Check sheet for the modelled part. Datum: model origin and axes. Units: mm. A direction names the side the tool comes from. Coordinates: 2 decimals unless noted, no trailing zeros. Loops run counter-clockwise (first coordinate to the right, second up) from the corner with the lowest first, then second, coordinate; pieces in that order, holes last. Notation, with made-up numbers: M -40,13.25 L -4,13.25 A28 ccw -4,45.25 Z; hole C 62,19 d1. An arc over 180 degrees is marked long. Write each question's results on one line, items separated by ' | '. Start each with the question number.
from build123d import *

# Parameters (mm, degrees)
PAD_DEPTH         = 10
SKETCH001_W       = 20.5
SKETCH001_H       = 6.5
POCKET_DEPTH      = 8
SKETCH002_W       = 20.5
SKETCH002_H       = 4
POCKET001_DEPTH   = 5
POCKET002_DEPTH   = 5
POCKET002_FACE1_W = 10
POCKET002_FACE1_H = 34
PAD001_DEPTH      = 1
PAD001_FACE3_W    = 10
PAD001_FACE3_H    = 10
PAD002_DEPTH      = 1


with BuildPart() as part:
    # Sketch → Pad (new body)
    with BuildSketch(Plane.XZ):
        Polygon((0, 10), (24, 10), (24, 2), (34, 2), (34, 0), (0, 0), align=None)
    extrude(amount=PAD_DEPTH)

    # Sketch001 (on Face7 of Pad) → Pocket (cut)
    with BuildSketch(Plane(origin=(0, 0, 0), x_dir=(1, 0, 0), z_dir=(0, 1, 0))):
        with Locations((11.75, -5.25)):
            Rectangle(SKETCH001_W, SKETCH001_H)
    extrude(amount=-POCKET_DEPTH, mode=Mode.SUBTRACT)

    # Sketch002 (on Face13 of Pocket) → Pocket001 (cut)
    with BuildSketch(Plane(origin=(0, -8, 0), x_dir=(1, 0, 0), z_dir=(0, 1, 0))):
        with Locations((11.75, -5.25)):
            Rectangle(SKETCH002_W, SKETCH002_H)
    extrude(amount=-POCKET001_DEPTH, mode=Mode.SUBTRACT)

    # Sketch003 (on Face6 of Pocket001) → Pocket002 (cut)
    with BuildSketch(Plane(origin=(0, 0, 2), x_dir=(-1, 0, 0), z_dir=(0, 0, 1))):
        with BuildLine():
            ThreePointArc((-30, 4.05), (-31.55, 2.5), (-30, 0.95))
            Line((-30, 0.95), (-26, 0.95))
            ThreePointArc((-26, 0.95), (-24.45, 2.5), (-26, 4.05))
            Line((-26, 4.05), (-30, 4.05))
        make_face()
    extrude(amount=-POCKET002_DEPTH, mode=Mode.SUBTRACT)

    # Pocket002 Face1 → Pad001 (add)
    with BuildSketch(Plane(origin=(16.314411, -5.155816, 0), x_dir=(0, -1, 0), z_dir=(0, 0, -1))):
        with Locations((-0.155816, -0.685589)):
            Rectangle(POCKET002_FACE1_W, POCKET002_FACE1_H)
        with BuildLine():
            Line((-1.105816, -9.685589), (-1.105816, -13.685589))
            ThreePointArc((-1.105816, -13.685589), (-2.655816, -15.235589), (-4.205816, -13.685589))
            Line((-4.205816, -13.685589), (-4.205816, -9.685589))
            ThreePointArc((-4.205816, -9.685589), (-2.655816, -8.135589), (-1.105816, -9.685589))
        make_face(mode=Mode.SUBTRACT)
    extrude(amount=PAD001_DEPTH)

    # Pad001 Face3 → Pad002 (add)
    with BuildSketch(Plane(origin=(29.249183, -5.622957, 2), x_dir=(0, 1, 0), z_dir=(0, 0, 1))):
        with Locations((0.622957, 0.249183)):
            Rectangle(PAD001_FACE3_W, PAD001_FACE3_H)
        with BuildLine():
            ThreePointArc((4.672957, -0.750817), (3.122957, -2.300817), (1.572957, -0.750817))
            Line((1.572957, -0.750817), (1.572957, 3.249183))
            ThreePointArc((1.572957, 3.249183), (3.122957, 4.799183), (4.672957, 3.249183))
            Line((4.672957, 3.249183), (4.672957, -0.750817))
        make_face(mode=Mode.SUBTRACT)
    extrude(amount=PAD002_DEPTH)


solid = part.part
Item 1: Section check C-C (x = 16.5). Record the cut outline in (y, z), plus the area to 3 significant figures.
Item 2: Thickness scan on line 1 (Z direction, x = 5, y = -1.5); line 2 (X direction, y = -4.5, z = 6.25); line 3 (X direction, y = -6.5, z = 2.5). Record the ranges inside material, lowest first.
Item 3: Depth check by flat-ended pin: P1, Ø3, axis at x = 26.5, y = -2.5, coming from the +Z side; P2, Ø3.5, axis at y = -4, z = 8, coming from the +X side; P3, Ø1, axis at x = 25.5, y = -5, coming from the +Z side. Enter the tip coordinate at first touch or a pass-through.
Item 4: Section check B-B (z = 5). Record the cut outline in (x, y), plus the area to 3 significant figures.
Item 5: Tool access check on faces 1 (the face through (24, -5, 7)), 2 (the face through (12, -4, 8.5)), 3 (the face through (28, -0.95, 1)). Record the directions out of +Z, -Z, +X, -X, +Y, -Y that give a thin tool (end or side, any length) a straight path to the whole face; none if there is none.
Item 6: Section check D-D (y = -8.75). Record the cut outline in (x, z).
Item 7: Section check A-A (y = -2.5). Record the cut outline in (x, z).
Item 8: Release check for a two-part mould opening along X. For faces 4 (the face through (0, -5, 5)), 5 (the face through (28, -4.05, 1)), 6 (the face through (17, -5, -1)) record: +X half, -X half, draft (parallel to the pull), parting line (faces both ways), or undercut.
Computed values:
1) outline: M -10,-1 L 0,-1 L 0,2 L -8,2 L -8,3.25 L -10,3.25 Z; M -10,7.25 L -8,7.25 L -8,8.5 L 0,8.5 L 0,10 L -10,10 Z | area: 50.0 mm²
2) line 1: z = -1 to 2, 8.5 to 10 | line 2: x = 0 to 1.5, 22 to 24 | line 3: x = 0 to 1.5, 22 to 34
3) P1: passes through | P2: stops at x = 24 | P3: stops at z = 3
4) outline: M 0,-10 L 1.5,-10 L 1.5,0 L 0,0 Z; M 22,-10 L 24,-10 L 24,0 L 22,0 Z | area: 35.0 mm²
5) face 1: +Z, +X, +Y, -Y | face 2: +Y | face 3: +Z, -Z
6) outline: M 0,-1 L 34,-1 L 34,3 L 24,3 L 24,10 L 0,10 Z; hole M 1.5,3.25 L 22,3.25 L 22,7.25 L 1.5,7.25 Z
7) outline: M 0,-1 L 24.45,-1 L 24.45,3 L 24,3 L 24,10 L 0,10 Z; M 31.55,-1 L 34,-1 L 34,3 L 31.55,3 Z; hole M 1.5,2 L 22,2 L 22,8.5 L 1.5,8.5 Z
8) face 4: -X half | face 5: undercut | face 6: draft
